```python
from build123d import *

# Parameters (mm, degrees)
EXTRUDE_1_DEPTH          = 12.375
EXTRUDE_1_DEPTH_BACK     = 3
SKETCH_1_R               = 13
CUT_EXTRUDE_1_DEPTH      = 20
CUT_EXTRUDE_1_DEPTH_BACK = 10
SKETCH_2_R               = 10.5
SWEEP_1_PITCH            = 5.5


with BuildPart() as part:
    # 草图1 → 凸台-拉伸1 (new, two sides: drawn at the far end of the back side and taken through both)
    with BuildSketch(Plane.XY.offset(-EXTRUDE_1_DEPTH_BACK)):
        Circle(SKETCH_1_R)
    extrude(amount=EXTRUDE_1_DEPTH + EXTRUDE_1_DEPTH_BACK)

    # 草图2 → 切除-拉伸1 (cut, two sides: drawn at the far end of the back side and taken through both)
    with BuildSketch(Plane.XY.offset(-CUT_EXTRUDE_1_DEPTH_BACK)):
        Circle(SKETCH_2_R)
    extrude(amount=CUT_EXTRUDE_1_DEPTH + CUT_EXTRUDE_1_DEPTH_BACK, mode=Mode.SUBTRACT)

    # 扫描1: the profile of 草图4 screwed along a right-hand helix of 2.25 turns, 14 arcs to a turn; built about Z, then put on its axis
    sweep_1_z = Axis((0, 0, 0), (0, 0, 1))
    sweep_1_corners = [(10.5, 0, 0), (10.5, 0.249236025, -2.989628974), (8.5, 0.207696687, -2.491357479), (8.5, 0.041539337, -0.498271496)]
    with BuildLine(mode=Mode.PRIVATE) as sweep_1_profile:
        Line(sweep_1_corners[0], sweep_1_corners[1])
        Line(sweep_1_corners[1], sweep_1_corners[2])
        Line(sweep_1_corners[2], sweep_1_corners[3])
        Line(sweep_1_corners[3], sweep_1_corners[0])
    sweep_1_cap = Face(sweep_1_profile.wire())
    sweep_1_turn_angles = [0, 12.857142857, 25.714285714, 38.571428571, 51.428571429, 64.285714286, 77.142857143, 90, 102.857142857, 115.714285714, 128.571428571, 141.428571429, 154.285714286, 167.142857143, 180, 192.857142857, 205.714285714, 218.571428571, 231.428571429, 244.285714286, 257.142857143, 270, 282.857142857, 295.714285714, 308.571428571, 321.428571429, 334.285714286, 347.142857143, 360]
    sweep_1_turn_weights = [1, 0.9749279121818236, 1, 0.9749279121818236, 1, 0.9749279121818236, 1, 0.9749279121818236, 1, 0.9749279121818236, 1, 0.9749279121818236, 1, 0.9749279121818236, 1, 0.9749279121818236, 1, 0.9749279121818236, 1, 0.9749279121818236, 1, 0.9749279121818236, 1, 0.9749279121818237, 1, 0.9749279121818236, 1, 0.9749279121818236, 1]
    sweep_1_turn_rails = [Edge.make_bspline([Vector(p[0], p[1], 0).rotate(sweep_1_z, sweep_1_turn_angles[k]) / sweep_1_turn_weights[k] + Vector(0, 0, p[2] + SWEEP_1_PITCH * sweep_1_turn_angles[k] / 360) for k in range(29)], [0, 0, 0, 1, 1, 2, 2, 3, 3, 4, 4, 5, 5, 6, 6, 7, 7, 8, 8, 9, 9, 10, 10, 11, 11, 12, 12, 13, 13, 14, 14, 14], 2, sweep_1_turn_weights) for p in sweep_1_corners]
    sweep_1_turn_sides = [Face.make_surface_from_curves(sweep_1_turn_rails[p[0]], sweep_1_turn_rails[p[1]]) for p in [(0, 1), (1, 2), (2, 3), (3, 0)]]
    sweep_1_last_angles = [720, 732.857142857, 745.714285714, 758.571428571, 771.428571429, 784.285714286, 797.142857143, 803.571428571, 810]
    sweep_1_last_weights = [1, 0.9749279121818237, 1, 0.9749279121818235, 1, 0.9749279121818237, 1, 0.9937122098932412, 1]
    sweep_1_last_rails = [Edge.make_bspline([Vector(p[0], p[1], 0).rotate(sweep_1_z, sweep_1_last_angles[k]) / sweep_1_last_weights[k] + Vector(0, 0, p[2] + SWEEP_1_PITCH * sweep_1_last_angles[k] / 360) for k in range(9)], [0, 0, 0, 1, 1, 2, 2, 3, 3, 4, 4, 4], 2, sweep_1_last_weights) for p in sweep_1_corners]
    sweep_1_last_sides = [Face.make_surface_from_curves(sweep_1_last_rails[p[0]], sweep_1_last_rails[p[1]]) for p in [(0, 1), (1, 2), (2, 3), (3, 0)]]
    sweep_1 = Plane(origin=(0, 0, 0), x_dir=(-0.7071067811865414, -0.7071067811865537, 0), z_dir=(0, 0, 1)) * Solid(Shell([*[p.moved(Location((0, 0, SWEEP_1_PITCH * i))) for i in range(2) for p in sweep_1_turn_sides], *sweep_1_last_sides, sweep_1_cap, sweep_1_cap.rotate(sweep_1_z, 810).moved(Location((0, 0, SWEEP_1_PITCH * 810 / 360)))]))
    add(sweep_1)


solid = part.part
```
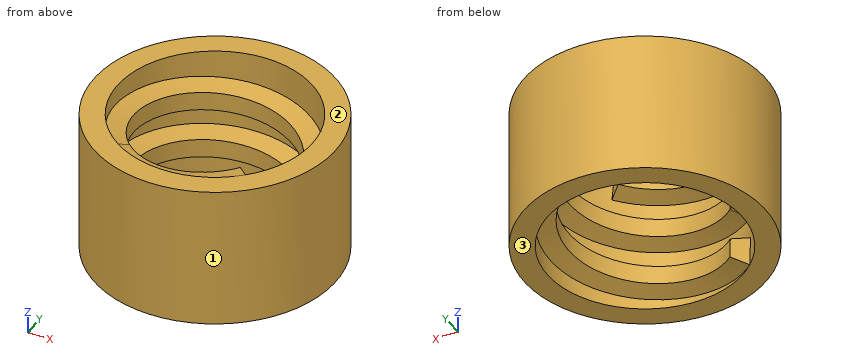
Build history of the part. All positions in model axes, mm. Face numbers are marked on the shaded views. Round coordinates to 2 decimals unless told otherwise and drop trailing zeros. Write each loop counter-clockwise with the first axis right and the second up, starting at its lowest first coordinate (ties: lowest second). Pieces come first, ordered by that corner, then holes.
1) Drill centre lines: probe 1 along Y at (x, z) = (0, 7.5); probe 2 along Y at (x, z) = (0, 9.75); probe 3 along X at (y, z) = (-3.75, 5.25). Where is each one in solid material? Low to high.
2) Mould opens along Z. For the marked faces 1, 2 and 3 say: +Z half, -Z half, draft (parallel to the pull), parting line (faces both ways), or undercut.
3) Pin check, flat tips, straight feed: pin 1 (1 mm diameter, centred on x = -8.5, z = 8.5, fed in from +Y); pin 2 (12.5 mm diameter, centred on x = 0, y = 0, fed in from +Z); pin 3 (5 mm diameter, centred on y = 5.5, z = 7.5, fed in from +X); pin 4 (2 mm diameter, centred on y = 3.5, z = 3.5, fed in from +X). Stop position of each tip, or through.
4) Band-saw the part on A-A, the plane y = -11. List the corners of the cut face in (x, z) (3 decimals).
Ans:
1. probe 1: y = -13 to -10.5, 8.5 to 13
1. probe 2: y = -13 to -8.5, 10.5 to 13
1. probe 3: x = -12.45 to -9.81, 7.63 to 12.45
2. face 1: draft
2. face 2: +Z half
2. face 3: -Z half
3. pin 1: stops at y = 10.25
3. pin 2: passes through
3. pin 3: stops at x = 12.65
3. pin 4: stops at x = 12.76
4. outline: (-6.928, -3) - (6.928, -3) - (6.928, 12.375) - (-6.928, 12.375) - close
